For this review, take the finished solid that the model builds, in its own axes (mm). A direction names the side the tool comes from. Round coordinates to 2 decimals unless told otherwise and drop trailing zeros. Order: outer loops, then holes, each group sorted by start corner. A loop starts at its lowest first (then second) coordinate and runs counter-clockwise, first axis right, second up. Notation, with made-up numbers: M 69.5,72.25 L 95.5,72.25 A20 cw 95.5,107.25 Z; hole C 73.25,89.25 d8. An arc over 180 degrees is marked long. Answer as a JSON object with one key per item and string values.
from build123d import *

# Parameters (mm, degrees)
SALIENTE_EXTRUIR1_DEPTH  = 3
CROQUIS2_W               = 50
CROQUIS2_H               = 25
SALIENTE_EXTRUIR2_DEPTH  = 165
CROQUIS5_W               = 20
CROQUIS5_H               = 165
CROQUIS5_W_2             = 1.746423124
CROQUIS5_H_2             = 0.642620727
CORTAR_EXTRUIR2_DEPTH    = 76
REDONDEO1_R              = 10
CROQUIS8_W               = 50
CROQUIS8_H               = 19.339026843
SALIENTE_EXTRUIR10_DEPTH = 60
CROQUIS12_W              = 46
CROQUIS12_H              = 15.339026843
CORTAR_EXTRUIR6_DEPTH    = 60
REDONDEO5_R              = 1.25
CROQUIS15_W              = 46
CROQUIS15_H              = 60
CORTAR_EXTRUIR7_DEPTH    = 2
CROQUIS16_R              = 2
CROQUIS16_W              = 19.3
CROQUIS16_H              = 29.3
CORTAR_EXTRUIR8_DEPTH    = 12


with BuildPart() as part:
    # Croquis1 → Saliente-Extruir1 (new body)
    with BuildSketch(Plane(origin=(0, 0, 0), x_dir=(1, 0, 0), z_dir=(0, 1, 0))):
        Polygon((-46, 21.805695142), (-46, -21.805695142), (-21.805695142, -46), (21.805695142, -46), (46, -21.805695142), (46, 21.805695142), (21.805695142, 46), (-21.805695142, 46), align=None)
    extrude(amount=SALIENTE_EXTRUIR1_DEPTH)

    # Croquis2 → Saliente-Extruir2 (add)
    with BuildSketch(Plane(origin=(0, 3, 0), x_dir=(1, 0, 0), z_dir=(0, 1, 0))):
        Rectangle(CROQUIS2_W, CROQUIS2_H)
    extrude(amount=SALIENTE_EXTRUIR2_DEPTH)

    # Croquis5 → Cortar-Extruir2 (cut)
    with BuildSketch(Plane.ZY.offset(25)):
        with Locations((2.5, 85.5)):
            Rectangle(CROQUIS5_W, CROQUIS5_H)
        with Locations((-13.373211562, 137.85800573)):
            Rectangle(CROQUIS5_W_2, CROQUIS5_H_2)
    extrude(amount=-CORTAR_EXTRUIR2_DEPTH, mode=Mode.SUBTRACT)

    # Redondeo1
    redondeo1_edges = [part.edges().sort_by_distance(p)[0] for p in [
        (-25, 168, -10),
        (25, 168, -10),
    ]]
    fillet(redondeo1_edges, radius=REDONDEO1_R)

    # Croquis8 → Saliente-Extruir10 (add)
    with BuildSketch(Plane(origin=(0, 3, -4.577154817), x_dir=(1, 0, 0), z_dir=(0, 1, 0))):
        with Locations((0.044911917, -6.746668238)):
            Rectangle(CROQUIS8_W, CROQUIS8_H)
    extrude(amount=SALIENTE_EXTRUIR10_DEPTH)

    # Croquis12 → Cortar-Extruir6 (cut)
    with BuildSketch(Plane(origin=(0, 63, 0), x_dir=(1, 0, 0), z_dir=(0, 1, 0))):
        with Locations((0.044911917, -2.169513422)):
            Rectangle(CROQUIS12_W, CROQUIS12_H)
    extrude(amount=-CORTAR_EXTRUIR6_DEPTH, mode=Mode.SUBTRACT)

    # Redondeo5
    redondeo5_edges = [part.edges().sort_by_distance(p)[0] for p in [
        (-24.955088083, 33, 11.839026843),
        (25.044911917, 33, 11.839026843),
    ]]
    fillet(redondeo5_edges, radius=REDONDEO5_R)

    # Croquis15 → Cortar-Extruir7 (cut)
    with BuildSketch(Plane.XY.offset(-5.5)):
        with Locations((0.044911917, 33)):
            Rectangle(CROQUIS15_W, CROQUIS15_H)
    extrude(amount=-CORTAR_EXTRUIR7_DEPTH, mode=Mode.SUBTRACT)

    # Croquis16 → Cortar-Extruir8 (cut)
    with BuildSketch(Plane(origin=(0, 3, 0), x_dir=(1, 0, 0), z_dir=(0, 1, 0))):
        with Locations(Location((-17, 29, 0), (0, 0, 270))):
            Circle(CROQUIS16_R)
        with Locations(Location((16.4, 29, 0), (0, 0, 270))):
            Circle(CROQUIS16_R)
        with Locations(Location((-16, -29, 0), (0, 0, 270))):
            Circle(CROQUIS16_R)
        with Locations(Location((16, -29, 0), (0, 0, 270))):
            Circle(CROQUIS16_R)
        with Locations((0, 31.35)):
            Rectangle(CROQUIS16_W, CROQUIS16_H)
        with Locations((0, -31.35)):
            Rectangle(CROQUIS16_W, CROQUIS16_H)
    extrude(amount=-CORTAR_EXTRUIR8_DEPTH, mode=Mode.SUBTRACT)


solid = part.part
1) Add section D-D on y = 137. State the section outline as (x, z) points.
Geometry check:
{"outline": "M -25,-12.5 L 25,-12.5 L 25,-7.5 L -25,-7.5 Z"}
2) Add section A-A on x = 6.5. State the section outline as (y, z) points.
Geometry check:
{"outline": "M 0,-16.7 L 3,-16.7 L 3,-12.5 L 168,-12.5 L 168,-7.5 L 3,-7.5 L 3,9.84 L 63,9.84 L 63,11.84 L 3,11.84 L 3,16.7 L 0,16.7 Z"}
3) Mouldability with a two-part tool opening along X and no side actions: class faces 4 (the flat face through (-33.733, 1.479, -34.072)), 5 (the cylindrical face through (21.99, 165.15, -10.04)), 6 (the flat face through (-22.955, 33, 1)) as +X half, -X half, draft (parallel to the pull), parting line (faces both ways), or undercut.
Geometry check:
{"face 4": "-X half", "face 5": "+X half", "face 6": "undercut"}
4) Machinability: for faces 1 (the flat face through (0, 84, -12.5)), 2 (the flat face through (0, 33, 11.839)), 3 (the flat face through (23.045, 33, 1)), which of the approach directions +Z, -Z, +X, -X, +Y, -Y give a long, thin tool a straight path to every point of the face, cutting with its end or side? Answer none if there is none.
Geometry check:
{"face 1": "-Z, +X, -X, +Y", "face 2": "+Z, +X, -X, +Y", "face 3": "+Y"}
5) Add section B-B on z = -5. State the section outline as (x, y) points.
Geometry check:
{"outline": "M -46,0 L 46,0 L 46,3 L 25.04,3 L 25.04,63 L 23.04,63 L 23.04,3 L -22.96,3 L -22.96,63 L -24.96,63 L -24.96,3 L -46,3 Z"}
6) For L1, parallel to Z at x = -2, y = 51; L2, parallel to X at y = 2.45, z = -29; L3, parallel to Z at x = 15, y = 118, list the stretches that pass through material, from the lowest coordinate up.
Geometry check:
{"L1": "z = -12.5 to -7.5, 9.84 to 11.84", "L2": "x = -38.81 to -19, -15 to -9.65, 9.65 to 14.4, 18.4 to 38.81", "L3": "z = -12.5 to -7.5"}
7) Add section C-C on z = 29. State the section outline as (x, y) points.
Geometry check:
{"outline": "M -38.81,0 L -18,0 L -18,3 L -38.81,3 Z; M -14,0 L -9.65,0 L -9.65,3 L -14,3 Z; M 9.65,0 L 14,0 L 14,3 L 9.65,3 Z; M 18,0 L 38.81,0 L 38.81,3 L 18,3 Z"}
8) Insertion check: P1, Ø4, axis at y = 51, z = -11, coming from the +X side; P2, Ø15, axis at x = -5.5, y = 100, coming from the +Z side; P3, Ø9, axis at y = 47, z = -1.5, coming from the -X side. Each pin has a flat end and moves straight along its axis. Give the tip position at first contact, or say it passes through.
Geometry check:
{"P1": "stops at x = 25", "P2": "stops at z = -7.5", "P3": "stops at x = -24.96"}
